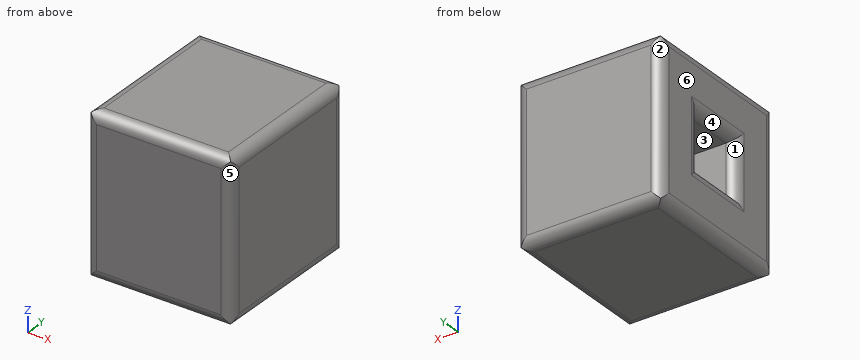
```python
from build123d import *

# Parameters (mm, degrees)
F0_W         = 76.2
F0_H         = 76.2
F1_DEPTH     = 69.85
F2_T         = -25.4
F3_R         = 5.08
F4_R         = 5.08
F5_T1_DEPTH  = 91.44
F5_T3_DEPTH  = 25.4
F5_T5_DEPTH  = 25.4
F5_T11_DEPTH = 38.1
F5_T15_DEPTH = 38.1
F5_T22_DEPTH = 38.1
F5_T26_DEPTH = 38.1
F5_T33_DEPTH = 38.1
F5_T37_DEPTH = 38.1
F5_T44_DEPTH = 38.1
F5_T48_DEPTH = 38.1
F6_T1_DEPTH  = 91.44


# Not quite as in the source:
# - a fillet or chamfer that OpenCascade refuses, or shapes differently, is made with other operations: its cross-section is extruded or revolved along the edge and cut away or added


with BuildPart() as f1:
    # F0 (on Right) → F1 (new body)
    with BuildSketch(Plane.YZ):
        Rectangle(F0_W, F0_H)
    extrude(amount=F1_DEPTH)

    # F2
    f2_openings = [f1.faces().sort_by_distance(p)[0] for p in [
        (0, 0, 0),
    ]]
    offset(amount=F2_T, openings=f2_openings)

    # F3
    f3_edges = [f1.edges().sort_by_distance(p)[0] for p in [
        (34.925, 38.1, -38.1),
        (34.925, 38.1, 38.1),
        (0, 38.1, 0),
        (69.85, 38.1, 0),
    ]]
    fillet(f3_edges, radius=F3_R)

    # F4
    f4_edges = [f1.edges().sort_by_distance(p)[0] for p in [
        (34.925, -38.1, 38.1),
        (34.925, -38.1, -38.1),
        (0, -38.1, 0),
        (69.85, -38.1, 0),
    ]]
    fillet(f4_edges, radius=F4_R)

    # F5: fillet of radius 5.08 on 8 edges, made by hand

    # F5_s2 → F5_t1 (cut)
    with BuildSketch(Plane.XZ.offset(-45.72)):
        with BuildLine():
            ThreePointArc((5.08, -38.1), (1.4878975516, -36.6121024484), (0, -33.02))
            Line((0, -33.02), (0, -38.1))
            Line((0, -38.1), (5.08, -38.1))
        make_face()
        with BuildLine():
            ThreePointArc((0, 33.02), (1.4878975516, 36.6121024484), (5.08, 38.1))
            Line((5.08, 38.1), (0, 38.1))
            Line((0, 38.1), (0, 33.02))
        make_face()
    extrude(amount=F5_T1_DEPTH, mode=Mode.SUBTRACT)

    # F5_s4 → F5_t3 (cut)
    with BuildSketch(Plane.XY.offset(-12.7)):
        with BuildLine():
            ThreePointArc((0, -17.78), (1.4878975516, -14.1878975516), (5.08, -12.7))
            Line((5.08, -12.7), (0, -12.7))
            Line((0, -12.7), (0, -17.78))
        make_face()
        with BuildLine():
            ThreePointArc((0, 17.78), (1.4878975516, 14.1878975516), (5.08, 12.7))
            Line((5.08, 12.7), (0, 12.7))
            Line((0, 12.7), (0, 17.78))
        make_face()
    extrude(amount=F5_T3_DEPTH, mode=Mode.SUBTRACT)

    # F5_s6 → F5_t5 (cut)
    with BuildSketch(Plane.XZ.offset(-12.7)):
        with BuildLine():
            ThreePointArc((0, 17.78), (1.4878975516, 14.1878975516), (5.08, 12.7))
            Line((5.08, 12.7), (0, 12.7))
            Line((0, 12.7), (0, 17.78))
        make_face()
        with BuildLine():
            ThreePointArc((0, -17.78), (1.4878975516, -14.1878975516), (5.08, -12.7))
            Line((5.08, -12.7), (0, -12.7))
            Line((0, -12.7), (0, -17.78))
        make_face()
    extrude(amount=F5_T5_DEPTH, mode=Mode.SUBTRACT)


with BuildPart() as f5_tool9:
    # F5_s10 → F5_t11 (new body)
    with BuildSketch(Plane.XY.offset(25.4)):
        with BuildLine():
            ThreePointArc((0, -17.78), (1.4878975516, -14.1878975516), (5.08, -12.7))
            Line((5.08, -12.7), (0, -12.7))
            Line((0, -12.7), (0, -17.78))
        make_face()
    extrude(amount=-F5_T11_DEPTH)

    split(bisect_by=Plane.XY.offset(12.7), keep=Keep.TOP)


with BuildPart() as f5_tool13:
    # F5_s14 → F5_t15 (new body)
    with BuildSketch(Plane.XZ.offset(-12.7)):
        with BuildLine():
            ThreePointArc((0, 17.78), (1.4878975516, 14.1878975516), (5.08, 12.7))
            Line((5.08, 12.7), (0, 12.7))
            Line((0, 12.7), (0, 17.78))
        make_face()
    extrude(amount=F5_T15_DEPTH)

    split(bisect_by=Plane.XZ.offset(12.7), keep=Keep.TOP)


with BuildPart() as f5_tool9_1:
    add(f5_tool9.part)

    # F5_t17: intersect F5_tool13
    add(f5_tool13.part, mode=Mode.INTERSECT)


with BuildPart() as f1_1:
    add(f1.part)

    # F5_t7: cut F5_tool9
    add(f5_tool9_1.part, mode=Mode.SUBTRACT)


with BuildPart() as f5_tool20:
    # F5_s21 → F5_t22 (new body)
    with BuildSketch(Plane.XY.offset(12.7)):
        with BuildLine():
            ThreePointArc((0, -17.78), (1.4878975516, -14.1878975516), (5.08, -12.7))
            Line((5.08, -12.7), (0, -12.7))
            Line((0, -12.7), (0, -17.78))
        make_face()
    extrude(amount=-F5_T22_DEPTH)

    split(bisect_by=Plane.XY.offset(-12.7), keep=Keep.BOTTOM)


with BuildPart() as f5_tool24:
    # F5_s25 → F5_t26 (new body)
    with BuildSketch(Plane.XZ.offset(25.4)):
        with BuildLine():
            ThreePointArc((0, -17.78), (1.4878975516, -14.1878975516), (5.08, -12.7))
            Line((5.08, -12.7), (0, -12.7))
            Line((0, -12.7), (0, -17.78))
        make_face()
    extrude(amount=-F5_T26_DEPTH)

    split(bisect_by=Plane.XZ.offset(12.7), keep=Keep.TOP)


with BuildPart() as f5_tool20_1:
    add(f5_tool20.part)

    # F5_t28: intersect F5_tool24
    add(f5_tool24.part, mode=Mode.INTERSECT)


with BuildPart() as f1_2:
    add(f1_1.part)

    # F5_t18: cut F5_tool20
    add(f5_tool20_1.part, mode=Mode.SUBTRACT)


with BuildPart() as f5_tool31:
    # F5_s32 → F5_t33 (new body)
    with BuildSketch(Plane.XZ.offset(-25.4)):
        with BuildLine():
            ThreePointArc((0, 17.78), (1.4878975516, 14.1878975516), (5.08, 12.7))
            Line((5.08, 12.7), (0, 12.7))
            Line((0, 12.7), (0, 17.78))
        make_face()
    extrude(amount=F5_T33_DEPTH)

    split(bisect_by=Plane.XZ.offset(-12.7), keep=Keep.BOTTOM)


with BuildPart() as f5_tool35:
    # F5_s36 → F5_t37 (new body)
    with BuildSketch(Plane.XY.offset(-12.7)):
        with BuildLine():
            ThreePointArc((0, 17.78), (1.4878975516, 14.1878975516), (5.08, 12.7))
            Line((5.08, 12.7), (0, 12.7))
            Line((0, 12.7), (0, 17.78))
        make_face()
    extrude(amount=F5_T37_DEPTH)

    split(bisect_by=Plane.XY.offset(12.7), keep=Keep.TOP)


with BuildPart() as f5_tool31_1:
    add(f5_tool31.part)

    # F5_t39: intersect F5_tool35
    add(f5_tool35.part, mode=Mode.INTERSECT)


with BuildPart() as f1_3:
    add(f1_2.part)

    # F5_t29: cut F5_tool31
    add(f5_tool31_1.part, mode=Mode.SUBTRACT)


with BuildPart() as f5_tool42:
    # F5_s43 → F5_t44 (new body)
    with BuildSketch(Plane.XY.offset(-25.4)):
        with BuildLine():
            ThreePointArc((0, 17.78), (1.4878975516, 14.1878975516), (5.08, 12.7))
            Line((5.08, 12.7), (0, 12.7))
            Line((0, 12.7), (0, 17.78))
        make_face()
    extrude(amount=F5_T44_DEPTH)

    split(bisect_by=Plane.XY.offset(-12.7), keep=Keep.BOTTOM)


with BuildPart() as f5_tool46:
    # F5_s47 → F5_t48 (new body)
    with BuildSketch(Plane.XZ.offset(12.7)):
        with BuildLine():
            ThreePointArc((0, -17.78), (1.4878975516, -14.1878975516), (5.08, -12.7))
            Line((5.08, -12.7), (0, -12.7))
            Line((0, -12.7), (0, -17.78))
        make_face()
    extrude(amount=-F5_T48_DEPTH)

    split(bisect_by=Plane.XZ.offset(-12.7), keep=Keep.BOTTOM)


with BuildPart() as f5_tool42_1:
    add(f5_tool42.part)

    # F5_t50: intersect F5_tool46
    add(f5_tool46.part, mode=Mode.INTERSECT)


with BuildPart() as f1_4:
    add(f1_3.part)

    # F5_t40: cut F5_tool42
    add(f5_tool42_1.part, mode=Mode.SUBTRACT)

    # F6: fillet of radius 5.08 on 4 edges, made by hand

    # F6_s2 → F6_t1 (cut)
    with BuildSketch(Plane.XZ.offset(-45.72)):
        with BuildLine():
            ThreePointArc((64.77, -38.1), (68.3621024484, -36.6121024484), (69.85, -33.02))
            Line((69.85, -33.02), (69.85, -38.1))
            Line((69.85, -38.1), (64.77, -38.1))
        make_face()
        with BuildLine():
            ThreePointArc((64.77, 38.1), (68.3621024484, 36.6121024484), (69.85, 33.02))
            Line((69.85, 33.02), (69.85, 38.1))
            Line((69.85, 38.1), (64.77, 38.1))
        make_face()
    extrude(amount=F6_T1_DEPTH, mode=Mode.SUBTRACT)


solid = f1_4.part
```
Geometry check sheet. Reference: the model listing, model coordinates, mm. Face numbers are marked on the shaded views. A direction names the side the tool comes from. Coordinates: 2 decimals unless noted, no trailing zeros. Write each loop counter-clockwise with the first axis right and the second up, starting at its lowest first coordinate (ties: lowest second). Pieces come first, ordered by that corner, then holes. Notation, with made-up numbers: M -20,-23 L 34,-23 A27 ccw 34,8 Z; hole C 50,-34 d8. An arc over 180 degrees is marked long. Use one line per item in the form item = value. Start each with the question number.
1) Set-up check for the marked faces 1 and 2: record each of +Z, -Z, +X, -X, +Y, -Y from which the full face is reachable in a straight line by a thin tool's end or side.
2) Go/stop test with flat-tipped pins: pin 1 Ø10 at (y, z) = (5, -7) entering from -X; pin 2 Ø12 at (y, z) = (11, 3.5) entering from -X. Record where each tip stops, or that it passes through.
3) Release check for a two-part mould opening along Y. For the marked faces 3, 4, 5 and 6 record: pulls with the +Y half, pulls with the -Y half, needs draft (parallel to the pull), parting line crosses it, or undercut.
4) Thickness scan on probe 1 along Z at (x, y) = (25.5, 5); probe 2 along Y at (x, z) = (13, -34.5). Record the ranges inside material, lowest first. Write a range as from..to.
5) Section check A-A on x = 38. Enter the section's corners in (y, z), and give its area (3 significant figures).
6) Section check B-B on y = -4.5. Enter the section's corners in (x, z), and give its area (3 significant figures).
Responses:
q1.face_1 = -X
q1.face_2 = +Z, -Z, -X, +Y
q2.pin_1 = 44.45
q2.pin_2 = 0.06
q3.face_3 = undercut
q3.face_4 = undercut
q3.face_5 = pulls with the -Y half
q3.face_6 = needs draft
q4.probe_1 = -38.1..-12.7, 12.7..38.1
q4.probe_2 = -37.88..37.88
q5.outline = M -38.1,-33.02 A5.08 ccw -33.02,-38.1 L 33.02,-38.1 A5.08 ccw 38.1,-33.02 L 38.1,33.02 A5.08 ccw 33.02,38.1 L -33.02,38.1 A5.08 ccw -38.1,33.02 Z; hole M -12.7,-12.7 L 12.7,-12.7 L 12.7,12.7 L -12.7,12.7 Z
q5.area = 5,140 mm2
q6.outline = M 0,-33.02 A5.08 ccw 5.08,-38.1 L 64.77,-38.1 A5.08 ccw 69.85,-33.02 L 69.85,33.02 A5.08 ccw 64.77,38.1 L 5.08,38.1 A5.08 ccw 0,33.02 L 0,17.78 A5.08 ccw 5.08,12.7 L 44.45,12.7 L 44.45,-12.7 L 5.08,-12.7 A5.08 ccw 0,-17.78 Z
q6.area = 4,160 mm2
